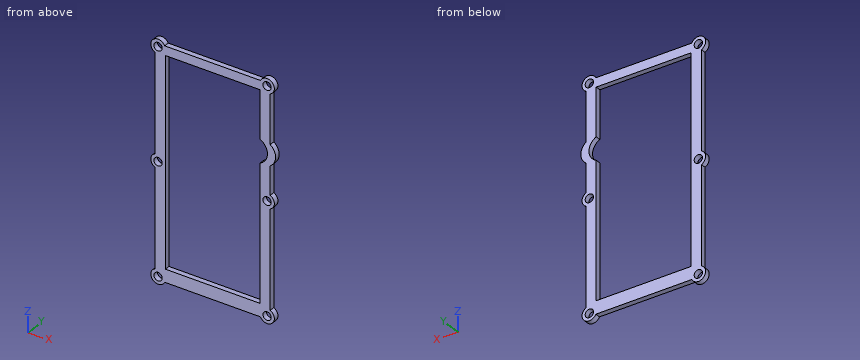
from build123d import *

# Parameters (mm, degrees)
F0_R     = 4
F1_DEPTH = 2.5


with BuildPart() as f1:
    # F0 (on Front) → F1 (new body, symmetric)
    with BuildSketch(Plane.XZ):
        with BuildLine():
            Line((-57.774334, -17.846146), (-57.774334, -112.197036))
            ThreePointArc((-57.774334, -112.197036), (-59.724081, -123.471338), (-48.449779, -121.521591))
            Line((-48.449779, -121.521591), (43.901111, -121.521591))
            ThreePointArc((43.901111, -121.521591), (55.175413, -123.471338), (53.225666, -112.197036))
            Line((53.225666, -112.197036), (53.225666, -17.846146))
            ThreePointArc((53.225666, -17.846146), (57.225666, -11.521591), (53.225666, -5.197036))
            Line((53.225666, -5.197036), (53.225666, 22.303822))
            ThreePointArc((53.225666, 22.303822), (58.408131, 32.160811), (53.225666, 42.017801))
            Line((53.225666, 42.017801), (53.225666, 89.153854))
            ThreePointArc((53.225666, 89.153854), (55.175413, 100.428157), (43.901111, 98.478409))
            Line((43.901111, 98.478409), (-48.449779, 98.478409))
            ThreePointArc((-48.449779, 98.478409), (-59.724081, 100.428157), (-57.774334, 89.153854))
            Line((-57.774334, 89.153854), (-57.774334, -5.197036))
            ThreePointArc((-57.774334, -5.197036), (-61.774334, -11.521591), (-57.774334, -17.846146))
        make_face()
        with Locations((-54.774334, -118.521591)):
            Circle(F0_R, mode=Mode.SUBTRACT)
        with Locations((50.225666, -118.521591)):
            Circle(F0_R, mode=Mode.SUBTRACT)
        with Locations((-54.774334, -11.521591)):
            Circle(F0_R, mode=Mode.SUBTRACT)
        with Locations((-54.774334, 95.478409)):
            Circle(F0_R, mode=Mode.SUBTRACT)
        with BuildLine():
            Line((-47.672213, -109.113894), (-47.672213, 89.714533))
            Line((-47.672213, 89.714533), (43.570419, 89.714533))
            Line((43.570419, 89.714533), (43.570419, 43.387121))
            ThreePointArc((43.570419, 43.387121), (50.570419, 32.478409), (43.570419, 21.569697))
            Line((43.570419, 21.569697), (43.570419, -109.113894))
            Line((43.570419, -109.113894), (-47.672213, -109.113894))
        make_face(mode=Mode.SUBTRACT)
        with Locations((50.225666, -11.521591)):
            Circle(F0_R, mode=Mode.SUBTRACT)
        with Locations((50.225666, 95.478409)):
            Circle(F0_R, mode=Mode.SUBTRACT)
    extrude(amount=F1_DEPTH, both=True)


solid = f1.part
Design review of the part built by this model. Coordinates are the model's own, in mm. Coordinates: 2 decimals unless noted, no trailing zeros. Loops run counter-clockwise (first coordinate to the right, second up) from the corner with the lowest first, then second, coordinate; pieces in that order, holes last. Notation, with made-up numbers: (-2, -8) -> (25, -8) arc R6 cw to (25, -3) -> close; hole circle Ø5 at (0, 89.25). An arc over 180 degrees is marked (long way). Use a Markdown table: item, result. Add a question column.
Item 1: Clearance check with flat-ended pins moving along their axes: P1, Ø2.5, axis at y = 0.5, z = 74, coming from the +X side; P2, Ø2.5, axis at x = 11, y = 0, coming from the -Z side; P3, Ø2, axis at x = -4, y = 0, coming from the +Z side; P4, Ø6.5, axis at x = -54.77, z = -11.52, coming from the +Y side. State where each tip first meets the part, or that it passes through.
Item 2: Wall thickness on L1, parallel to Z at x = 29, y = 1.6; L2, parallel to X at y = 0.75, z = -50; L3, parallel to X at y = 1.1, z = 33: over which ranges is each line inside the solid? List them lowest first. Write a range as from..to.
Item 3: We need section C-C, the plane y = 1.2. Write out the cut boundary in (x, z).
Item 4: We need section A-A, the plane x = 39. Write out the cut boundary in (y, z).
Item 5: We need section B-B, the plane z = 56. Write out the cut boundary in (x, y), and give its area (3 significant figures).
Numbers:
| question | item | result |
|---|---|---|
| 1 | P1 | stops at x = 53.23 |
| 1 | P2 | stops at z = -121.52 |
| 1 | P3 | stops at z = 98.48 |
| 1 | P4 | passes through |
| 2 | L1 | z = -121.52..-109.11, 89.71..98.48 |
| 2 | L2 | x = -57.77..-47.67, 43.57..53.23 |
| 2 | L3 | x = -57.77..-47.67, 50.56..58.38 |
| 3 | outline | (-57.77, -112.2) arc R7 ccw (long way) to (-48.45, -121.52) -> (43.9, -121.52) arc R7 ccw (long way) to (53.23, -112.2) -> (53.23, -17.85) arc R7 ccw to (53.23, -5.2) -> (53.23, 22.3) arc R11.97 ccw to (53.23, 42.02) -> (53.23, 89.15) arc R7 ccw (long way) to (43.9, 98.48) -> (-48.45, 98.48) arc R7 ccw (long way) to (-57.77, 89.15) -> (-57.77, -5.2) arc R7 ccw to (-57.77, -17.85) -> close; hole circle Ø8 at (-54.77, -118.52); hole circle Ø8 at (-54.77, -11.52); hole circle Ø8 at (-54.77, 95.48); hole (-47.67, -109.11) -> (43.57, -109.11) -> (43.57, 21.57) arc R12 ccw to (43.57, 43.39) -> (43.57, 89.71) -> (-47.67, 89.71) -> close; hole circle Ø8 at (50.23, -118.52); hole circle Ø8 at (50.23, -11.52); hole circle Ø8 at (50.23, 95.48) |
| 4 | outline | (-2.5, -121.52) -> (2.5, -121.52) -> (2.5, -109.11) -> (-2.5, -109.11) -> close; (-2.5, 89.71) -> (2.5, 89.71) -> (2.5, 98.48) -> (-2.5, 98.48) -> close |
| 5 | outline | (-57.77, -2.5) -> (-47.67, -2.5) -> (-47.67, 2.5) -> (-57.77, 2.5) -> close; (43.57, -2.5) -> (53.23, -2.5) -> (53.23, 2.5) -> (43.57, 2.5) -> close |
| 5 | area | 98.8 mm^2 |
